Part model, mm, in its own coordinate system. Give positions to 0.01 mm unless a question says otherwise; leave off trailing zeros.
from build123d import *

# Parameters (mm, degrees)
SKETCH1_R      = 3.302
EXTRUDE1_DEPTH = 762


with BuildPart() as part:
    # Sketch1 → Extrude1 (new body)
    with BuildSketch(Plane.XY):
        with BuildLine():
            Line((4.699, 19.05), (17.78, 19.05))
            Line((17.78, 19.05), (19.05, 17.78))
            Line((19.05, 17.78), (19.05, 4.699))
            ThreePointArc((19.05, 4.699), (18.901210245, 4.339789755), (18.542, 4.191))
            Line((18.542, 4.191), (15.24, 4.191))
            ThreePointArc((15.24, 4.191), (14.880789755, 4.339789755), (14.732, 4.699))
            Line((14.732, 4.699), (14.732, 6.223))
            ThreePointArc((14.732, 6.223), (14.880789755, 6.582210245), (15.24, 6.731))
            Line((15.24, 6.731), (16.002, 6.731))
            ThreePointArc((16.002, 6.731), (16.361210245, 6.879789755), (16.51, 7.239))
            Line((16.51, 7.239), (16.51, 8.1534))
            ThreePointArc((16.51, 8.1534), (16.361210245, 8.512610245), (16.002, 8.6614))
            Line((16.002, 8.6614), (10.667871762, 8.6614))
            ThreePointArc((10.667871762, 8.6614), (10.473468578, 8.622730803), (10.308661517, 8.512610245))
            Line((10.308661517, 8.512610245), (5.842, 4.045948728))
            Line((5.842, 4.045948728), (5.842, -4.045948728))
            Line((5.842, -4.045948728), (10.308661517, -8.512610245))
            ThreePointArc((10.308661517, -8.512610245), (10.473468578, -8.622730803), (10.667871762, -8.6614))
            Line((10.667871762, -8.6614), (16.002, -8.6614))
            ThreePointArc((16.002, -8.6614), (16.361210245, -8.512610245), (16.51, -8.1534))
            Line((16.51, -8.1534), (16.51, -7.239))
            ThreePointArc((16.51, -7.239), (16.361210245, -6.879789755), (16.002, -6.731))
            Line((16.002, -6.731), (15.24, -6.731))
            ThreePointArc((15.24, -6.731), (14.880789755, -6.582210245), (14.732, -6.223))
            Line((14.732, -6.223), (14.732, -4.699))
            ThreePointArc((14.732, -4.699), (14.880789755, -4.339789755), (15.24, -4.191))
            Line((15.24, -4.191), (18.542, -4.191))
            ThreePointArc((18.542, -4.191), (18.901210245, -4.339789755), (19.05, -4.699))
            Line((19.05, -4.699), (19.05, -17.78))
            Line((19.05, -17.78), (17.78, -19.05))
            Line((17.78, -19.05), (4.699, -19.05))
            ThreePointArc((4.699, -19.05), (4.339789755, -18.901210245), (4.191, -18.542))
            Line((4.191, -18.542), (4.191, -15.24))
            ThreePointArc((4.191, -15.24), (4.339789755, -14.880789755), (4.699, -14.732))
            Line((4.699, -14.732), (6.223, -14.732))
            ThreePointArc((6.223, -14.732), (6.582210245, -14.880789755), (6.731, -15.24))
            Line((6.731, -15.24), (6.731, -16.002))
            ThreePointArc((6.731, -16.002), (6.879789755, -16.361210245), (7.239, -16.51))
            Line((7.239, -16.51), (8.1534, -16.51))
            ThreePointArc((8.1534, -16.51), (8.512610245, -16.361210245), (8.6614, -16.002))
            Line((8.6614, -16.002), (8.6614, -10.667871762))
            ThreePointArc((8.6614, -10.667871762), (8.622730803, -10.473468578), (8.512610245, -10.308661517))
            Line((8.512610245, -10.308661517), (4.045948728, -5.842))
            Line((4.045948728, -5.842), (-4.045948728, -5.842))
            Line((-4.045948728, -5.842), (-8.512610245, -10.308661517))
            ThreePointArc((-8.512610245, -10.308661517), (-8.622730803, -10.473468578), (-8.6614, -10.667871762))
            Line((-8.6614, -10.667871762), (-8.6614, -16.002))
            ThreePointArc((-8.6614, -16.002), (-8.512610245, -16.361210245), (-8.1534, -16.51))
            Line((-8.1534, -16.51), (-7.239, -16.51))
            ThreePointArc((-7.239, -16.51), (-6.879789755, -16.361210245), (-6.731, -16.002))
            Line((-6.731, -16.002), (-6.731, -15.24))
            ThreePointArc((-6.731, -15.24), (-6.582210245, -14.880789755), (-6.223, -14.732))
            Line((-6.223, -14.732), (-4.699, -14.732))
            ThreePointArc((-4.699, -14.732), (-4.339789755, -14.880789755), (-4.191, -15.24))
            Line((-4.191, -15.24), (-4.191, -18.542))
            ThreePointArc((-4.191, -18.542), (-4.339789755, -18.901210245), (-4.699, -19.05))
            Line((-4.699, -19.05), (-17.78, -19.05))
            Line((-17.78, -19.05), (-19.05, -17.78))
            Line((-19.05, -17.78), (-19.05, -4.699))
            ThreePointArc((-19.05, -4.699), (-18.901210245, -4.339789755), (-18.542, -4.191))
            Line((-18.542, -4.191), (-15.24, -4.191))
            ThreePointArc((-15.24, -4.191), (-14.880789755, -4.339789755), (-14.732, -4.699))
            Line((-14.732, -4.699), (-14.732, -6.223))
            ThreePointArc((-14.732, -6.223), (-14.880789755, -6.582210245), (-15.24, -6.731))
            Line((-15.24, -6.731), (-16.002, -6.731))
            ThreePointArc((-16.002, -6.731), (-16.361210245, -6.879789755), (-16.51, -7.239))
            Line((-16.51, -7.239), (-16.51, -8.1534))
            ThreePointArc((-16.51, -8.1534), (-16.361210245, -8.512610245), (-16.002, -8.6614))
            Line((-16.002, -8.6614), (-10.667871762, -8.6614))
            ThreePointArc((-10.667871762, -8.6614), (-10.473468578, -8.622730803), (-10.308661517, -8.512610245))
            Line((-10.308661517, -8.512610245), (-5.842, -4.045948728))
            Line((-5.842, -4.045948728), (-5.842, 4.045948728))
            Line((-5.842, 4.045948728), (-10.308661517, 8.512610245))
            ThreePointArc((-10.308661517, 8.512610245), (-10.473468578, 8.622730803), (-10.667871762, 8.6614))
            Line((-10.667871762, 8.6614), (-16.002, 8.6614))
            ThreePointArc((-16.002, 8.6614), (-16.361210245, 8.512610245), (-16.51, 8.1534))
            Line((-16.51, 8.1534), (-16.51, 7.239))
            ThreePointArc((-16.51, 7.239), (-16.361210245, 6.879789755), (-16.002, 6.731))
            Line((-16.002, 6.731), (-15.24, 6.731))
            ThreePointArc((-15.24, 6.731), (-14.880789755, 6.582210245), (-14.732, 6.223))
            Line((-14.732, 6.223), (-14.732, 4.699))
            ThreePointArc((-14.732, 4.699), (-14.880789755, 4.339789755), (-15.24, 4.191))
            Line((-15.24, 4.191), (-18.542, 4.191))
            ThreePointArc((-18.542, 4.191), (-18.901210245, 4.339789755), (-19.05, 4.699))
            Line((-19.05, 4.699), (-19.05, 17.78))
            Line((-19.05, 17.78), (-17.78, 19.05))
            Line((-17.78, 19.05), (-4.699, 19.05))
            ThreePointArc((-4.699, 19.05), (-4.339789755, 18.901210245), (-4.191, 18.542))
            Line((-4.191, 18.542), (-4.191, 15.24))
            ThreePointArc((-4.191, 15.24), (-4.339789755, 14.880789755), (-4.699, 14.732))
            Line((-4.699, 14.732), (-6.223, 14.732))
            ThreePointArc((-6.223, 14.732), (-6.582210245, 14.880789755), (-6.731, 15.24))
            Line((-6.731, 15.24), (-6.731, 16.002))
            ThreePointArc((-6.731, 16.002), (-6.879789755, 16.361210245), (-7.239, 16.51))
            Line((-7.239, 16.51), (-8.1534, 16.51))
            ThreePointArc((-8.1534, 16.51), (-8.512610245, 16.361210245), (-8.6614, 16.002))
            Line((-8.6614, 16.002), (-8.6614, 10.667871762))
            ThreePointArc((-8.6614, 10.667871762), (-8.622730803, 10.473468578), (-8.512610245, 10.308661517))
            Line((-8.512610245, 10.308661517), (-4.045948728, 5.842))
            Line((-4.045948728, 5.842), (4.045948728, 5.842))
            Line((4.045948728, 5.842), (8.512610245, 10.308661517))
            ThreePointArc((8.512610245, 10.308661517), (8.622730803, 10.473468578), (8.6614, 10.667871762))
            Line((8.6614, 10.667871762), (8.6614, 16.002))
            ThreePointArc((8.6614, 16.002), (8.512610245, 16.361210245), (8.1534, 16.51))
            Line((8.1534, 16.51), (7.239, 16.51))
            ThreePointArc((7.239, 16.51), (6.879789755, 16.361210245), (6.731, 16.002))
            Line((6.731, 16.002), (6.731, 15.24))
            ThreePointArc((6.731, 15.24), (6.582210245, 14.880789755), (6.223, 14.732))
            Line((6.223, 14.732), (4.699, 14.732))
            ThreePointArc((4.699, 14.732), (4.339789755, 14.880789755), (4.191, 15.24))
            Line((4.191, 15.24), (4.191, 18.542))
            ThreePointArc((4.191, 18.542), (4.339789755, 18.901210245), (4.699, 19.05))
        make_face()
        Circle(SKETCH1_R, mode=Mode.SUBTRACT)
        with BuildLine():
            Line((11.2014, 16.002), (11.2014, 11.7094))
            ThreePointArc((11.2014, 11.7094), (11.350189755, 11.350189755), (11.7094, 11.2014))
            Line((11.7094, 11.2014), (16.002, 11.2014))
            ThreePointArc((16.002, 11.2014), (16.361210245, 11.350189755), (16.51, 11.7094))
            Line((16.51, 11.7094), (16.51, 16.002))
            ThreePointArc((16.51, 16.002), (16.361210245, 16.361210245), (16.002, 16.51))
            Line((16.002, 16.51), (11.7094, 16.51))
            ThreePointArc((11.7094, 16.51), (11.350189755, 16.361210245), (11.2014, 16.002))
        make_face(mode=Mode.SUBTRACT)
        with BuildLine():
            Line((-16.002, 11.2014), (-11.7094, 11.2014))
            ThreePointArc((-11.7094, 11.2014), (-11.350189755, 11.350189755), (-11.2014, 11.7094))
            Line((-11.2014, 11.7094), (-11.2014, 16.002))
            ThreePointArc((-11.2014, 16.002), (-11.350189755, 16.361210245), (-11.7094, 16.51))
            Line((-11.7094, 16.51), (-16.002, 16.51))
            ThreePointArc((-16.002, 16.51), (-16.361210245, 16.361210245), (-16.51, 16.002))
            Line((-16.51, 16.002), (-16.51, 11.7094))
            ThreePointArc((-16.51, 11.7094), (-16.361210245, 11.350189755), (-16.002, 11.2014))
        make_face(mode=Mode.SUBTRACT)
        with BuildLine():
            Line((-11.2014, -16.002), (-11.2014, -11.7094))
            ThreePointArc((-11.2014, -11.7094), (-11.350189755, -11.350189755), (-11.7094, -11.2014))
            Line((-11.7094, -11.2014), (-16.002, -11.2014))
            ThreePointArc((-16.002, -11.2014), (-16.361210245, -11.350189755), (-16.51, -11.7094))
            Line((-16.51, -11.7094), (-16.51, -16.002))
            ThreePointArc((-16.51, -16.002), (-16.361210245, -16.361210245), (-16.002, -16.51))
            Line((-16.002, -16.51), (-11.7094, -16.51))
            ThreePointArc((-11.7094, -16.51), (-11.350189755, -16.361210245), (-11.2014, -16.002))
        make_face(mode=Mode.SUBTRACT)
        with BuildLine():
            Line((16.002, -11.2014), (11.7094, -11.2014))
            ThreePointArc((11.7094, -11.2014), (11.350189755, -11.350189755), (11.2014, -11.7094))
            Line((11.2014, -11.7094), (11.2014, -16.002))
            ThreePointArc((11.2014, -16.002), (11.350189755, -16.361210245), (11.7094, -16.51))
            Line((11.7094, -16.51), (16.002, -16.51))
            ThreePointArc((16.002, -16.51), (16.361210245, -16.361210245), (16.51, -16.002))
            Line((16.51, -16.002), (16.51, -11.7094))
            ThreePointArc((16.51, -11.7094), (16.361210245, -11.350189755), (16.002, -11.2014))
        make_face(mode=Mode.SUBTRACT)
    extrude(amount=EXTRUDE1_DEPTH)


solid = part.part
Item 1: Drop flat-ended pins along their axis: P1, Ø3, axis at x = 2, z = 292.5, coming from the +Y side; P2, Ø2.5, axis at y = 2, z = 455.5, coming from the -X side. Give the stop position or say it passes through.
Item 2: Band-saw the part on A-A on z = 214. Give the number of separate pieces and of enclosed holes in the cut face, plus the area to 3 significant figures.
Item 3: Drill centre lines: probe 1 along Y at (x, z) = (13, 452); probe 2 along Y at (x, z) = (-4.5, 219); probe 3 along Y at (x, z) = (16, 697). Where is each one in solid material? Low to high.
Working result:
1. P1: stops at y = 5.84
1. P2: stops at x = -5.84
2. separate pieces: 1
2. enclosed holes: 5
2. area: 599 mm2
3. probe 1: y = -19.05 to -16.51, -11.2 to -8.66, 8.66 to 11.2, 16.51 to 19.05
3. probe 2: y = -19.01 to -14.77, -6.3 to 6.3, 14.77 to 19.01
3. probe 3: y = -19.05 to -16.51, -11.2 to -8.66, -6.73 to -4.19, 4.19 to 6.73, 8.66 to 11.2, 16.51 to 19.05
